CAD build for the part. Positions are in the model's coordinates, mm. A direction names the side the tool comes from. Coordinates: 2 decimals unless noted, no trailing zeros. Order: outer loops, then holes, each group sorted by start corner. A loop starts at its lowest first (then second) coordinate and runs counter-clockwise, first axis right, second up. Notation, with made-up numbers: (11.25, 64) - (58.25, 64) arc R23 ccw to (58.25, 84) - close; hole circle Ø11 at (38, 66.25). An arc over 180 degrees is marked (long way). Write each question's results on one line, items separated by ' | '. Start each with the question number.
Q1. Pin check, flat tips, straight feed: P1, Ø1.5, axis at x = -129, y = -49.5, coming from the -Z side; P2, Ø1.5, axis at x = -144.5, z = 1.5, coming from the +Y side; P3, Ø1, axis at x = -68, z = 1.5, coming from the -Y side. Stop position of each tip, or through.
Q2. Band-saw the part on D-D, the plane x = -95. Write the cut outline in (y, z), then the cut area to 3 significant figures.
Q3. Band-saw the part on C-C, the plane y = -79. Write the cut outline in (x, z), then the cut area to 3 significant figures.
Q4. Band-saw the part on A-A, the plane x = 11. Write the cut outline in (y, z).
Q5. Pull direction Y, two halves, no side cores. Call faces 1 (the flat face through (27.35, -171.934, 1.673)), 2 (the flat face through (-92, -133, 0)), 3 (the flat face through (114.404, -141.203, 1.627)): released by +Y, released by -Y, zero draft, split by the parting line, or undercut.
Q6. Band-saw the part on B-B, the plane z = 1.9. Count the separate pieces of the cut face and the enclosed holes in it, then the cut area to 3 significant figures.
Q7. Which spindle directions (+Z, -Z, +X, -X, +Y, -Y) get a long thin tool onto all of the face, cutting with end or side? Do faces 4 (the flat face through (-199.618, -66.097, 1.673)), 5 (the flat face through (-148.565, -238.528, 1.627)), 6 (the flat face through (124.574, -62.604, 1.627)). Say none if no direction does.
Q8. Wall check: probe 1 along X at (y, z) = (-119, 3.1); probe 2 along X at (y, z) = (-130.5, 2.45); probe 3 along X at (y, z) = (-105, 1.8). Give the ranges that are in metal, low to high.
```python
from build123d import *

# Parameters (mm, degrees)
SKETCH1_R           = 2
BOSS_EXTRUDE1_DEPTH = 3.3
SKETCH2_R           = 2
CUT_EXTRUDE1_DEPTH  = 463.683772706
CUT_EXTRUDE2_DEPTH  = 10
CUT_EXTRUDE3_DEPTH  = 10
SKETCH7_R           = 2
CUT_EXTRUDE4_DEPTH  = 10


with BuildPart() as part:
    # Sketch1 → Boss-Extrude1 (new body)
    with BuildSketch(Plane.XY):
        Polygon((-261.101380084, 0.003466677), (-110.332441909, 0.003466677), (-87.147938799, 49.722794044), (129.783117347, -51.433818728), (119.217660803, -74.091513404), (140.969047692, -84.234351686), (30.158539464, -321.868253447), (-332.364575351, -152.820948751), align=None)
        with Locations(Location((87.00354845, -69.000227384, 0), (0, 0, 180))):
            Circle(SKETCH1_R, mode=Mode.SUBTRACT)
        with Locations(Location((98.836859779, -43.623609347, 0), (0, 0, 180))):
            Circle(SKETCH1_R, mode=Mode.SUBTRACT)
        with Locations(Location((62.584548297, -26.718878877, 0), (0, 0, 180))):
            Circle(SKETCH1_R, mode=Mode.SUBTRACT)
        with Locations(Location((50.751236969, -52.095496914, 0), (0, 0, 180))):
            Circle(SKETCH1_R, mode=Mode.SUBTRACT)
        with Locations(Location((2.358593217, -286.837367237, 0), (0, 0, 180))):
            Circle(SKETCH1_R, mode=Mode.SUBTRACT)
        with Locations(Location((-306.422910118, -134.574853143, 0), (0, 0, 180))):
            Circle(SKETCH1_R, mode=Mode.SUBTRACT)
        with Locations(Location((20.484748958, -295.289732471, 0), (0, 0, 180))):
            Circle(SKETCH1_R, mode=Mode.SUBTRACT)
    extrude(amount=BOSS_EXTRUDE1_DEPTH)

    # Sketch2 → Cut-Extrude1 (cut, through all)
    with BuildSketch(Plane(origin=(0, 0, 0), x_dir=(-1, 0, 0), z_dir=(0, 0, -1))):
        with Locations((51.496578787, 22.064512657)):
            Circle(SKETCH2_R)
        with Locations((84.12365912, 37.27877008)):
            Circle(SKETCH2_R)
    extrude(amount=-CUT_EXTRUDE1_DEPTH, mode=Mode.SUBTRACT)

    # Sketch5 → Cut-Extrude2 (cut)
    with BuildSketch(Plane.XY.offset(3.3)):
        Polygon((65.954306233, -245.103983885), (-51.865706081, -190.163609859), (-30.734792994, -144.848220507), (87.08521932, -199.788594533), align=None)
    extrude(amount=-CUT_EXTRUDE2_DEPTH, mode=Mode.SUBTRACT)

    # Sketch6 → Cut-Extrude3 (cut)
    with BuildSketch(Plane.XY.offset(3.3)):
        Polygon((-178.748796266, -130.997053215), (-157.617883179, -85.681663863), (-242.810815161, -45.955547259), (-263.941728248, -91.270936611), align=None)
    extrude(amount=-CUT_EXTRUDE3_DEPTH, mode=Mode.SUBTRACT)

    # Sketch7 → Cut-Extrude4 (cut)
    with BuildSketch(Plane.XY.offset(3.3)):
        with Locations((-52.7985286, -172.571100935)):
            Circle(SKETCH7_R)
        with Locations((-44.346163365, -154.444945194)):
            Circle(SKETCH7_R)
        with Locations((-164.672545808, -120.403389962)):
            Circle(SKETCH7_R)
        with Locations((-156.220180573, -102.277234221)):
            Circle(SKETCH7_R)
    extrude(amount=-CUT_EXTRUDE4_DEPTH, mode=Mode.SUBTRACT)


solid = part.part
```
Results below:
1) P1: stops at z = 0 | P2: stops at y = 0 | P3: stops at y = -276.33
2) outline: (-263.51, 0) - (32.88, 0) - (32.88, 3.3) - (-263.51, 3.3) - close | area: 978 mm²
3) outline: (-297.94, 0) - (-258.22, 0) - (-258.22, 3.3) - (-297.94, 3.3) - close; (-171.95, 0) - (129.74, 0) - (129.74, 3.3) - (-171.95, 3.3) - close | area: 1,130 mm²
4) outline: (-312.93, 0) - (-219.48, 0) - (-219.48, 3.3) - (-312.93, 3.3) - close; (-164.31, 0) - (3.96, 0) - (3.96, 3.3) - (-164.31, 3.3) - close
5) face 1: undercut | face 2: zero draft | face 3: released by -Y
6) separate pieces: 1 | enclosed holes: 14 | area: 91,100 mm²
7) face 4: +Z, -Z | face 5: +Z, -Z, -X, -Y | face 6: +Z, -Z, +X
8) probe 1: x = -316.59 to -204.48, -173.15 to -166.1, -163.25 to 124.76 | probe 2: x = -321.96 to -179.81, -178.52 to 119.4 | probe 3: x = -310.07 to -234.5, -166.63 to 131.29
